Geometry check sheet. Reference: drawing and pictorial views, mm from the part's lowest x, y, z. A direction names the side the tool comes from. Round coordinates to 2 decimals unless told otherwise and drop trailing zeros. Write each loop counter-clockwise with the first axis right and the second up, starting at its lowest first coordinate (ties: lowest second). Pieces come first, ordered by that corner, then holes. Notation, with made-up numbers: (73.5, 14) -> (124.5, 14) arc R23 cw to (124.5, 42) -> close; hole circle Ø11 at (-0.75, 60.5). An arc over 180 degrees is marked (long way). Write item = value, one per line.
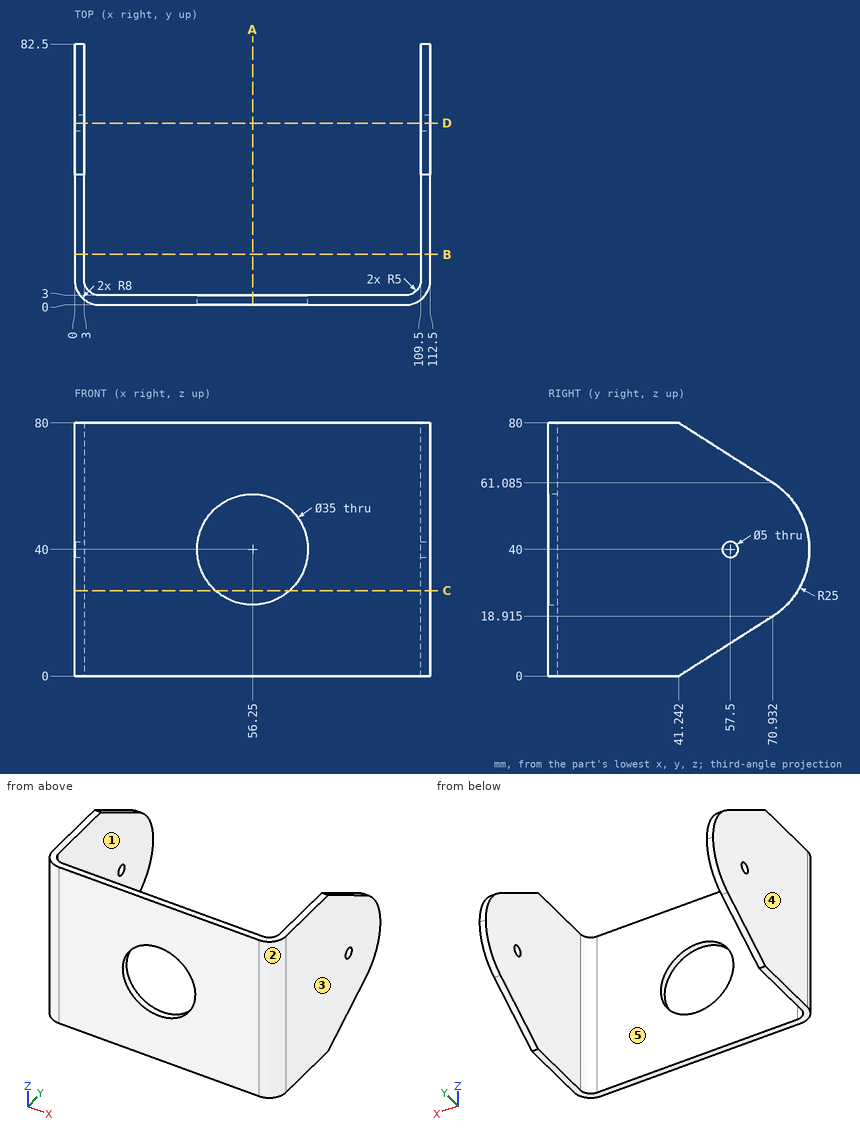
(1) Sectioned sample at D-D on y = 57.5. Enter the section's corners in (x, z).
Worked answers:
outline = (0, 10.36) -> (3, 10.36) -> (3, 37.5) -> (0, 37.5) -> close; (0, 42.5) -> (3, 42.5) -> (3, 69.64) -> (0, 69.64) -> close; (109.5, 10.36) -> (112.5, 10.36) -> (112.5, 37.5) -> (109.5, 37.5) -> close; (109.5, 42.5) -> (112.5, 42.5) -> (112.5, 69.64) -> (109.5, 69.64) -> close
(2) Access from +Z, -Z, +X, -X, +Y, -Y to the whole of each face (thin tool, end or side, straight path). Record for the marked faces 1 and 2.
Worked answers:
face_1 = +Z, -Z, +Y
face_2 = +Z, -Z, +X, -Y
(3) Sectioned sample at B-B on y = 16. Enter the section's corners in (x, z).
Worked answers:
outline = (0, 0) -> (3, 0) -> (3, 80) -> (0, 80) -> close; (109.5, 0) -> (112.5, 0) -> (112.5, 80) -> (109.5, 80) -> close
(4) Release check for a two-part mould opening along X. For the marked faces 3, 4 and 5 record: pulls with the +X half, pulls with the -X half, needs draft (parallel to the pull), parting line crosses it, or undercut.
Worked answers:
face_3 = pulls with the +X half
face_4 = pulls with the -X half
face_5 = undercut
(5) Material ranges on L1, parallel to X at y = 42, z = 33; L2, parallel to Y at x = 25, z = 64.5; L3, parallel to Z at x = 56, y = 1, recorded low to high. Write a range as [from, to].
Worked answers:
L1 = [0, 3], [109.5, 112.5]
L2 = [0, 3]
L3 = [0, 22.5], [57.5, 80]
(6) Sectioned sample at C-C on z = 27. Enter the section's corners in (x, y) (1 decimal).
Worked answers:
outline = (0, 8) arc R8 ccw to (8, 0) -> (44.5, 0) -> (44.5, 3) -> (8, 3) arc R5 cw to (3, 8) -> (3, 78.9) -> (0, 78.9) -> close; (68, 0) -> (104.5, 0) arc R8 ccw to (112.5, 8) -> (112.5, 78.9) -> (109.5, 78.9) -> (109.5, 8) arc R5 cw to (104.5, 3) -> (68, 3) -> close
(7) Sectioned sample at A-A on x = 56.25. Enter the section's corners in (y, z), then the cut area to 3 significant figures.
Worked answers:
outline = (0, 0) -> (3, 0) -> (3, 22.5) -> (0, 22.5) -> close; (0, 57.5) -> (3, 57.5) -> (3, 80) -> (0, 80) -> close
area = 135 mm²
(8) Go/stop test with flat-tipped pins: P1, Ø1, axis at x = 58, z = 25, coming from the +Y side; P2, Ø12, axis at x = 70, z = 72, coming from the +Y side. Record where each tip stops, or that it passes through.
Worked answers:
P1 = through
P2 = 3
